Build history of the part. All positions in model axes, mm. A direction names the side the tool comes from. Round coordinates to 2 decimals unless told otherwise and drop trailing zeros. Loops run counter-clockwise (first coordinate to the right, second up) from the corner with the lowest first, then second, coordinate; pieces in that order, holes last.
from build123d import *

# Parameters (mm, degrees)
F1_DEPTH = 63.5
F2_DEPTH = 25.4
F3_DEPTH = 7.9375
F5_R     = 6.35


with BuildPart() as f1:
    # F0 (on Front) → F1 (new body, symmetric)
    with BuildSketch(Plane.XZ):
        Polygon((22.225, 9.525), (-41.275, 9.525), (-41.275, -9.525), (41.275, -9.525), (41.275, 9.525), align=None)
    extrude(amount=F1_DEPTH, both=True)

    # F0 (on Front) → F2 (join, symmetric)
    with BuildSketch(Plane.XZ):
        with BuildLine():
            Line((22.225, 24.107097), (22.225, 9.525))
            Line((22.225, 9.525), (41.275, 9.525))
            Line((41.275, 9.525), (41.275, 24.107097))
            ThreePointArc((41.275, 24.107097), (45.92468, 35.332417), (57.15, 39.982097))
            Line((57.15, 39.982097), (60.657849, 39.982097))
            Line((60.657849, 39.982097), (60.657849, 59.032097))
            Line((60.657849, 59.032097), (57.15, 59.032097))
            add(Edge.make_bspline(
                [(54.762262, 58.950379), (55.554692, 58.980457), (56.350621, 59.007687), (57.15, 59.032097)],
                knots=[108.497511, 108.497511, 108.497511, 108.497511, 110.174558, 110.174558, 110.174558, 110.174558], degree=3))
            ThreePointArc((54.762262, 58.950379), (31.624059, 47.943664), (22.225, 24.107097))
        make_face()
    extrude(amount=F2_DEPTH, both=True)

    # F0 (on Front) → F3 (join, symmetric)
    with BuildSketch(Plane.XZ):
        with BuildLine():
            add(Edge.make_bspline(
                [(-41.275, 9.525), (-33.121447, 43.135956), (3.4956, 57.004461), (54.762262, 58.950379)],
                knots=[0, 0, 0, 0, 108.497511, 108.497511, 108.497511, 108.497511], degree=3))
            Line((-41.275, 9.525), (22.225, 9.525))
            Line((22.225, 9.525), (22.225, 24.107097))
            ThreePointArc((22.225, 24.107097), (31.624059, 47.943664), (54.762262, 58.950379))
        make_face()
    extrude(amount=F3_DEPTH, both=True)

    # F0 (on Front) → F4 (revolve)
    with BuildSketch(Plane.XZ):
        Polygon((60.657849, 65.545457), (60.657849, 59.032097), (101.433977, 59.032097), (101.6, 39.982097), (60.657849, 39.982097), (60.657849, 36.970457), (111.457849, 36.970457), (111.457849, 65.545457), align=None)
    revolve(axis=Axis((60.657849, 0, 51.257957), (0, 0, 1)))

    # F5
    f5_edges = [f1.edges().sort_by_distance(p)[0] for p in [
        (41.275, -63.5, 0),
        (-41.275, -63.5, 0),
        (41.275, 63.5, 0),
        (-41.275, 63.5, 0),
    ]]
    fillet(f5_edges, radius=F5_R)


solid = f1.part
(1) Slice it at C-C on y = -53. List the corners of the cut face in (x, z) (3 decimals).
Responses:
outline: (-41.275, -9.525) - (41.275, -9.525) - (41.275, 9.525) - (-41.275, 9.525) - close
(2) Which spindle directions (+Z, -Z, +X, -X, +Y, -Y) get a long thin tool onto all of the face, cutting with end or side? Do faces 1 (the face through (22.225, 17, 17)), 2 (the face through (-1, -7.938, 27)), 3 (the face through (109.1, 15.3, 51.5)), 4 (the face through (73, 1, 39.982)). Say none if no direction does.
Responses:
face 1: -X, +Y
face 2: -X, -Y
face 3: +Z
face 4: none
(3) Probe line 1 (Y direction, x = 59, z = 57.5); line 2 (Z direction, x = 86.5, y = 5); line 3 (Y direction, x = 33.5, z = 11.5). List the from-to ranges inside material, lowest first.
Responses:
line 1: y = -50.77 to -40.76, -25.4 to 25.4, 40.76 to 50.77
line 2: z = 36.97 to 39.98, 59.03 to 65.55
line 3: y = -25.4 to 25.4
(4) Slice it at B-B on y = 27.5. Count the separate pieces of the cut face and the enclosed holes in it, plus the area to 3 significant figures.
Responses:
separate pieces: 2
enclosed holes: 1
area: 2,860 mm2
(5) Pin check, flat tips, straight feed: P1, Ø10, axis at y = -20, z = 14.5, coming from the +X side (3 decimals); P2, Ø16, axis at y = 13, z = 19.5, coming from the -X side; P3, Ø15, axis at y = -12.5, z = 47, coming from the +X side; P4, Ø16, axis at y = -18, z = 15, coming from the -X side (3 decimals). Stop position of each tip, or through.
Responses:
P1: stops at x = 41.275
P2: stops at x = -40.21
P3: stops at x = 111.21
P4: stops at x = -41.275
(6) Pull direction Y, two halves, no side cores. Call faces 5 (the face through (60.658, 0, 49)), 6 (the face through (39.464, -61.59, 0.133)), 7 (the face through (24, 13, 39.982)), 8 (the face through (1, 35, 9.525)): +Y half, -Y half, draft (parallel to the pull), parting line (faces both ways), or undercut.
Responses:
face 5: undercut
face 6: -Y half
face 7: undercut
face 8: draft
(7) Slice it at A-A on z = 5. List the corners of the cut face in (x, y) (3 decimals), plus the area to 3 significant figures.
Responses:
outline: (-41.275, -57.15) arc R6.35 ccw to (-34.925, -63.5) - (34.925, -63.5) arc R6.35 ccw to (41.275, -57.15) - (41.275, 57.15) arc R6.35 ccw to (34.925, 63.5) - (-34.925, 63.5) arc R6.35 ccw to (-41.275, 57.15) - close
area: 10,400 mm2
